```python
from build123d import *

# Parameters (mm, degrees)
F2_DEPTH = 76.2
F3_R     = 5.08


# Not quite as in the source:
# - a feature names something its author has since deleted; it is built from what else it names


with BuildPart() as f2:
    # F1 (on offset) → F2 (new body)
    with BuildSketch(Plane.YZ.offset(76.2)):
        Polygon((0, -41.275), (0, 0), (-19.05, 0), (-19.05, -12.7), (-132.9298521399, -12.7), (-132.9298521399, -49.0773997059), align=None)
    extrude(amount=-F2_DEPTH)

    # F3
    f3_edges = [f2.edges().sort_by_distance(p)[0] for p in [
        (38.1, 0, -41.275),
        (76.2, 0, -20.6375),
        (0, 0, -20.6375),
        (76.2, -66.464926, -45.1762),
        (0, -66.464926, -45.1762),
        (0, -19.05, -6.35),
        (76.2, -19.05, -6.35),
        (0, -132.929852, -30.8887),
        (76.2, -132.929852, -30.8887),
        (38.1, -132.929852, -49.0774),
    ]]
    fillet(f3_edges, radius=F3_R)


solid = f2.part
```
Work out the finished part from the listing and answer in its coordinate system (mm). A direction names the side the tool comes from. Give positions to 0.01 mm unless a question says otherwise; leave off trailing zeros. Order: outer loops, then holes, each group sorted by start corner. A loop starts at its lowest first (then second) coordinate and runs counter-clockwise, first axis right, second up. Notation, with made-up numbers: M -8,78 L 28,78 A19 cw 28,87 Z; hole C -4,61.5 d6. An arc over 180 degrees is marked long. Return JSON: item names as keys, results as strings.
1) A tool of negligible diameter and unlimited length cuts with its end or side. For faces 1 (the cylindrical face through (1.528, -17.601, -6.439)), 2 (the flat face through (39, -19.05, -6)), 3 (the cylindrical face through (74.672, -1.449, -17.987)), 4 (the cylindrical face through (74.672, -17.601, -6.439)), from which of +Z, -Z, +X, -X, +Y, -Y can it reach the whole face along a straight path? Write none if from no direction.
Resolved:
{"face 1": "+Z, -X, -Y", "face 2": "+Z, +X, -X, -Y", "face 3": "+Z, -Z, +X, +Y", "face 4": "+Z, +X, -Y"}
2) Straight lines are drawn through the part: line 1 along Y through (x, z) = (47.5, -6.5); line 2 along Z through (x, y) = (43, -114); line 3 along Z through (x, y) = (5, -6). For each, find the intervals that lie inside material, in ascending order. Write a range as [from, to].
Resolved:
{"line 1": "[-19.05, 0]", "line 2": "[-47.97, -12.7]", "line 3": "[-41.63, 0]"}
3) Each of these flat-tipped pins is pushed along its axis until it touches: pin 1 (12 mm diameter, centred on x = 63, y = -108.5, fed in from +Z); pin 2 (6.5 mm diameter, centred on x = 47.5, z = -8, fed in from -Y); pin 3 (5 mm diameter, centred on y = -25, z = -42.5, fed in from +X). Where does it stop, or does it pass through?
Resolved:
{"pin 1": "z = -12.7", "pin 2": "y = -19.05", "pin 3": "x = 75.63"}
4) Section A-A, the plane z = -8 is taken. Write down the section's boundary in (x, y), plus the area to 3 significant figures.
Resolved:
{"outline": "M 0,-13.97 A5.08 ccw 5.08,-19.05 L 71.12,-19.05 A5.08 ccw 76.2,-13.97 L 76.2,-5.08 A5.08 ccw 71.12,0 L 5.08,0 A5.08 ccw 0,-5.08 Z", "area": "1,430 mm^2"}
5) Section B-B, the plane x = 52.5 is taken. Write down the section's boundary in (y, z).
Resolved:
{"outline": "M -132.93,-43.69 A5.08 ccw -127.55,-48.76 L -4.78,-41.56 A5.08 ccw 0,-36.48 L 0,0 L -19.05,0 L -19.05,-12.7 L -132.93,-12.7 Z"}
